Here's how the part is built. I have some questions about the finished solid (model axes, mm). A direction names the side the tool comes from. Coordinates: 2 decimals unless noted, no trailing zeros. Order: outer loops, then holes, each group sorted by start corner. A loop starts at its lowest first (then second) coordinate and runs counter-clockwise, first axis right, second up. Notation, with made-up numbers: (49, 74.25) - (59, 74.25) arc R15 cw to (59, 91.25) - close; hole circle Ø7 at (58, -4.5). An arc over 180 degrees is marked (long way). Use one line per item in the form item = value. Start each with the question number.
from build123d import *

# Parameters (mm, degrees)
SKETCH1_W           = 8
SKETCH1_H           = 3
BOSS_EXTRUDE1_DEPTH = 3
FILLET1_R           = 1
FILLET2_R           = 0.5


with BuildPart() as part:
    # Sketch1 → Boss-Extrude1 (new body)
    with BuildSketch(Plane(origin=(0, 0, 0), x_dir=(0, 0, -1), z_dir=(1, 0, 0))):
        Polygon((-5.6, 0), (-5.6, 3), (-6.75, 3), (-6.75, 5.4), (-5.6, 5.4), (-5.6, 10.4), (-2.4, 10.4), (-2.4, 5.4), (-1.25, 5.4), (-1.25, 3), (-2.4, 3), (-2.4, 0), (2.4, 0), (2.4, 3), (1.25, 3), (1.25, 5.4), (2.4, 5.4), (2.4, 10.4), (5.6, 10.4), (5.6, 5.4), (6.75, 5.4), (6.75, 3), (5.6, 3), (5.6, 0), (12.6, 0), (32.807259422, 35), (3.607259422, 35), (-16.6, 0), align=None)
        with Locations((15.320508076, 30)):
            Rectangle(SKETCH1_W, SKETCH1_H, mode=Mode.SUBTRACT)
    extrude(amount=BOSS_EXTRUDE1_DEPTH)

    # Fillet1
    fillet1_edges = [part.edges().sort_by_distance(p)[0] for p in [
        (1.5, 35, -3.607259422),
        (1.5, 35, -32.807259422),
    ]]
    fillet(fillet1_edges, radius=FILLET1_R)

    # Fillet2
    fillet2_edges = [part.edges().sort_by_distance(p)[0] for p in [
        (1.5, 0, 16.6),
        (1.5, 0, -12.6),
    ]]
    fillet(fillet2_edges, radius=FILLET2_R)


solid = part.part
1) Suppose I cut it at D-D, the plane z = -22. List the corners of the cut face in (x, y) for me.
2) Suppose I cut it at A-A, the plane z = -17. List the corners of the cut face in (x, y) for me, then the cut area to 3 significant figures.
3) I need wall thicknesses on probe 1 along Z at (x, y) = (1, 9.5); probe 2 along Z at (x, y) = (0.55, 5); probe 3 along Y at (x, z) = (2.1, -6.5). Which ranges of each line are inside material? Lowest first, please. Write a range as [from, to].
4) If we mould it in two halves opening along Y, with no side actions, what happens to faces 1 (the flat face through (1, 5.4, 2)), 2 (the flat face through (1, 5.4, -2)), 3 (the flat face through (1, 2, 2.4)), 4 (the flat face through (1, 35, -18))? For each: pulls with the +Y half, pulls with the -Y half, needs draft (parallel to the pull), parting line crosses it, or undercut.
5) Suppose I cut it at C-C, the plane y = 17. List the corners of the cut face in (x, z) for me, then the cut area to 3 significant figures.
6) Suppose I cut it at B-B, the plane y = 6. List the corners of the cut face in (x, z) for me.
7) For pin 1 (1.3 mm diameter, centred on x = 2, z = -2, fed in from -Y); pin 2 (1.2 mm diameter, centred on x = 1, y = 3.5, fed in from -Z); pin 3 (0.9 mm diameter, centred on x = 2, z = -13.5, fed in from -Y); pin 4 (0.9 mm diameter, centred on x = 1, y = 2, fed in from -Z), each with a flat end and sliding along its axis, tell me the tip position at first contact or that it passes through.
8) Which directions (+Z, -Z, +X, -X, +Y, -Y) give clear straight access to the entire face, cutting with the end or side of a thin tool? Please do faces 5 (the flat face through (1, 30, -19.321)), 6 (the flat face through (1, 0, 11)), 7 (the flat face through (1, 8, 2.4)).
From the geometry:
q1.outline = (0, 16.28) - (3, 16.28) - (3, 35) - (0, 35) - close
q2.outline = (0, 7.62) - (3, 7.62) - (3, 28.5) - (0, 28.5) - close; (0, 31.5) - (3, 31.5) - (3, 35) - (0, 35) - close
q2.area = 73.1 mm2
q3.probe_1 = [-18.08, -5.6], [-2.4, 2.4], [5.6, 11.12]
q3.probe_2 = [-15.49, -6.75], [-1.25, 1.25], [6.75, 13.71]
q3.probe_3 = [0, 3], [5.4, 35]
q4.face_1 = undercut
q4.face_2 = undercut
q4.face_3 = needs draft
q4.face_4 = pulls with the +Y half
q5.outline = (0, -22.41) - (3, -22.41) - (3, 6.79) - (0, 6.79) - close
q5.area = 87.6 mm2
q6.outline = (0, -16.06) - (3, -16.06) - (3, -5.6) - (0, -5.6) - close; (0, -2.4) - (3, -2.4) - (3, 2.4) - (0, 2.4) - close; (0, 5.6) - (3, 5.6) - (3, 13.14) - (0, 13.14) - close
q7.pin_1 = 0
q7.pin_2 = -14.97
q7.pin_3 = 0.78
q7.pin_4 = -14.01
q8.face_5 = +X, -X
q8.face_6 = +Z, -Z, +X, -X, -Y
q8.face_7 = +X, -X, -Y
